Part print with two shaded views. Sizes in mm from the minimum x, y, z corner. A direction names the side the tool comes from. Round coordinates to 2 decimals unless told otherwise and drop trailing zeros. Loops run counter-clockwise (first coordinate to the right, second up) from the corner with the lowest first, then second, coordinate; pieces in that order, holes last. Notation, with made-up numbers: (54.5, 20.25) - (98.5, 20.25) arc R30 ccw to (98.5, 49.25) - close; hole circle Ø10 at (6.5, -11.5). An arc over 180 degrees is marked (long way). One line per question, with ' | ' between items.
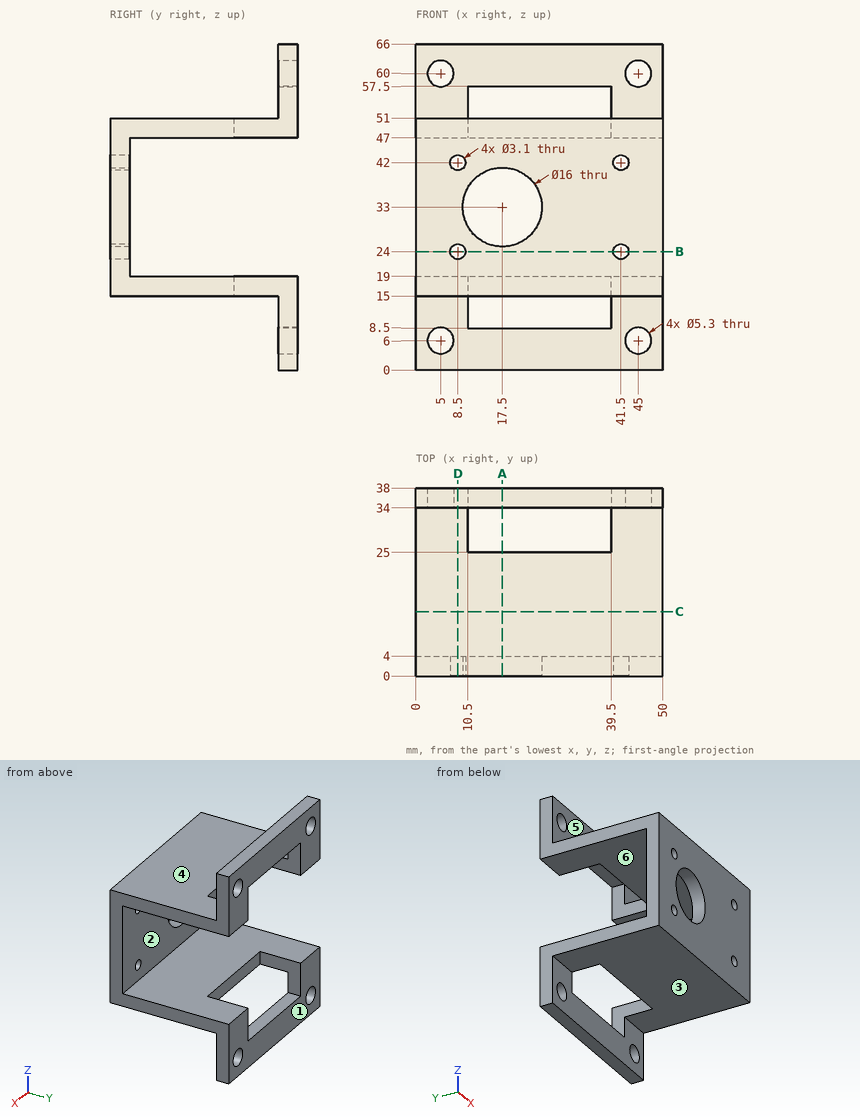
(1) Probe L1, parallel to X at y = 35.05, z = 6; L2, parallel to X at y = 1.7, z = 42; L3, parallel to Z at x = 18, y = 3. List the from-to ranges inside material, lowest first.
Results found:
L1: x = 0 to 2.35, 7.65 to 42.35, 47.65 to 50 | L2: x = 0 to 6.95, 10.05 to 39.95, 43.05 to 50 | L3: z = 15 to 25.02, 40.98 to 51
(2) Tool access for the marked faces 1, 2 and 3: list every direction of +Z, -Z, +X, -X, +Y, -Y with a clear straight run to the whole face (end or side of a thin tool).
Results found:
face 1: +Z, -Z, +X, -X, +Y | face 2: +X, -X, +Y | face 3: -Z, +X, -X, -Y
(3) Two-plate mould, pull along Z, no slides. Class the marked faces 4, 5 and 6: released by +Z, released by -Z, zero draft, split by the parting line, or undercut.
Results found:
face 4: released by +Z | face 5: zero draft | face 6: undercut
(4) Drop flat-ended pins along their axis: P1, Ø17, axis at x = 13.5, y = 15, coming from the +Z side; P2, Ø1.2, axis at x = 26.5, z = 49, coming from the +Y side; P3, Ø10, axis at x = 25, y = 18, coming from the -Z side. Give the stop position or say it passes through.
Results found:
P1: stops at z = 51 | P2: stops at y = 25 | P3: stops at z = 15
(5) Cut at B-B, the plane z = 24. Write the cut outline in (x, y).
Results found:
outline: (0, 0) - (6.95, 0) - (6.95, 4) - (0, 4) - close; (10.05, 0) - (39.95, 0) - (39.95, 4) - (10.05, 4) - close; (43.05, 0) - (50, 0) - (50, 4) - (43.05, 4) - close
(6) Cut at C-C, the plane y = 13. Write the cut outline in (x, z), then the cut area to 3 significant figures.
Results found:
outline: (0, 15) - (50, 15) - (50, 19) - (0, 19) - close; (0, 47) - (50, 47) - (50, 51) - (0, 51) - close | area: 400 mm²
(7) Cut at A-A, the plane x = 17.5. Write the cut outline in (y, z), then the cut area to 3 significant figures.
Results found:
outline: (0, 15) - (25, 15) - (25, 19) - (4, 19) - (4, 25) - (0, 25) - close; (0, 41) - (4, 41) - (4, 47) - (25, 47) - (25, 51) - (0, 51) - close; (34, 0) - (38, 0) - (38, 8.5) - (34, 8.5) - close; (34, 57.5) - (38, 57.5) - (38, 66) - (34, 66) - close | area: 316 mm²
(8) Cut at D-D, the plane x = 8.5. Write the cut outline in (y, z).
Results found:
outline: (0, 15) - (34, 15) - (34, 0) - (38, 0) - (38, 19) - (4, 19) - (4, 22.45) - (0, 22.45) - close; (0, 25.55) - (4, 25.55) - (4, 40.45) - (0, 40.45) - close; (0, 43.55) - (4, 43.55) - (4, 47) - (38, 47) - (38, 66) - (34, 66) - (34, 51) - (0, 51) - close
